Verification items for the finished model (mm, model axes). Face numbers are marked on the shaded views. A direction names the side the tool comes from. Coordinates: 2 decimals unless noted, no trailing zeros. Order: outer loops, then holes, each group sorted by start corner. A loop starts at its lowest first (then second) coordinate and runs counter-clockwise, first axis right, second up.
Q1. Depth check by flat-ended pin: P1, Ø8, axis at y = -13, z = 32, coming from the +X side; P2, Ø2, axis at x = 18.5, z = 22, coming from the -Y side; P3, Ø4, axis at y = 19, z = 17.5, coming from the -X side (3 decimals). Enter the tip coordinate at first touch or a pass-through.
Q2. Thickness scan on line 1 (X direction, y = 21.5, z = 8) (3 decimals); line 2 (Y direction, x = 17, z = 34.5); line 3 (Z direction, x = 84.5, y = -14) (3 decimals). Record the ranges inside material, lowest first.
Q3. Cross-section at A-A, the plane y = -52.5. Record the boundary of the cut face in (x, z) (3 decimals), and give its area (3 significant figures).
Q4. Set-up check for the marked faces 1, 2, 3 and 4: record each of +Z, -Z, +X, -X, +Y, -Y from which the full face is reachable in a straight line by a thin tool's end or side.
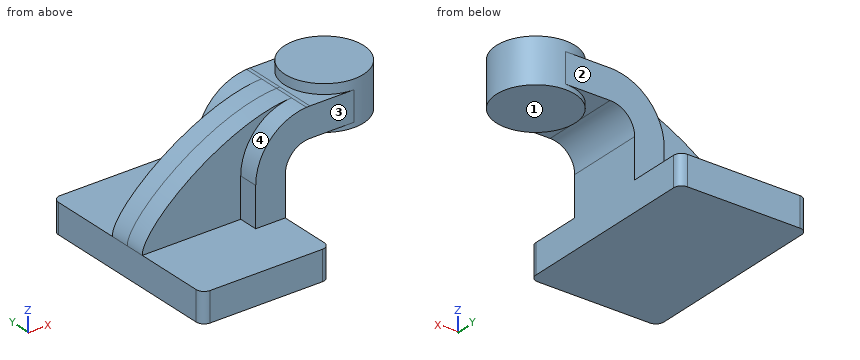
from build123d import *

# Parameters (mm, degrees)
F1_DEPTH = 63.5
F2_DEPTH = 25.4
F3_DEPTH = 12.7
F5_R     = 5.08


with BuildPart() as f1:
    # F0 (on Front) → F1 (new body, symmetric)
    with BuildSketch(Plane.XZ):
        Polygon((22.225, 9.525), (-41.275, 9.525), (-41.275, -9.525), (41.275, -9.525), (41.275, 9.525), align=None)
    extrude(amount=F1_DEPTH, both=True)

    # F0 (on Front) → F2 (join, symmetric)
    with BuildSketch(Plane.XZ):
        with BuildLine():
            Line((22.225, 34.925), (22.225, 9.525))
            Line((22.225, 9.525), (41.275, 9.525))
            Line((41.275, 9.525), (41.275, 34.925))
            ThreePointArc((41.275, 34.925), (45.92468, 46.15032), (57.15, 50.8))
            Line((57.15, 50.8), (60.325, 50.8))
            Line((60.325, 50.8), (60.325, 69.85))
            Line((60.325, 69.85), (57.15, 69.85))
            add(Edge.make_bspline(
                [(54.932606, 69.779538), (55.674519, 69.814721), (56.413753, 69.838317), (57.15, 69.85)],
                knots=[113.508266, 113.508266, 113.508266, 113.508266, 115.440834, 115.440834, 115.440834, 115.440834], degree=3))
            ThreePointArc((54.932606, 69.779538), (31.682392, 58.823882), (22.225, 34.925))
        make_face()
        Polygon((73.748745, 69.85), (60.325, 69.85), (60.325, 50.8), (73.748745, 50.8), (85.725, 50.8), (85.725, 61.9125), (85.725, 69.85), align=None)
    extrude(amount=F2_DEPTH, both=True)

    # F0 (on Front) → F3 (join, symmetric)
    with BuildSketch(Plane.XZ):
        with BuildLine():
            add(Edge.make_bspline(
                [(-41.275, 9.525), (-41.462009, 25.67143), (11.356779, 67.713042), (54.932606, 69.779538)],
                knots=[0, 0, 0, 0, 113.508266, 113.508266, 113.508266, 113.508266], degree=3))
            Line((-41.275, 9.525), (22.225, 9.525))
            Line((22.225, 9.525), (22.225, 34.925))
            ThreePointArc((22.225, 34.925), (31.682392, 58.823882), (54.932606, 69.779538))
        make_face()
    extrude(amount=F3_DEPTH, both=True)

    # F0 (on Front) → F4 (revolve)
    with BuildSketch(Plane.XZ):
        Polygon((111.125, 76.2), (85.725, 76.2), (85.725, 69.85), (85.725, 61.9125), (85.725, 50.8), (85.725, 47.625), (111.125, 47.625), align=None)
    revolve(axis=Axis((85.725, 0, 61.9125), (0, 0, 1)))

    # F5
    f5_edges = [f1.edges().sort_by_distance(p)[0] for p in [
        (-41.275, -63.5, 0),
        (41.275, -63.5, 0),
        (41.275, 63.5, 0),
        (-41.275, 63.5, 0),
    ]]
    fillet(f5_edges, radius=F5_R)


solid = f1.part
Check values:
1. P1: stops at x = 41.31
1. P2: stops at y = -12.7
1. P3: stops at x = 22.225
2. line 1: x = -41.275 to 41.275
2. line 2: y = -12.7 to 12.7
2. line 3: z = 47.625 to 76.2
3. outline: (-41.275, -9.525) - (41.275, -9.525) - (41.275, 9.525) - (-41.275, 9.525) - close
3. area: 1,570 mm2
4. face 1: -Z, +X, +Y, -Y
4. face 2: +Z, +X, -X, +Y
4. face 3: +Z, +X, -X, -Y
4. face 4: +Z, -X, -Y
